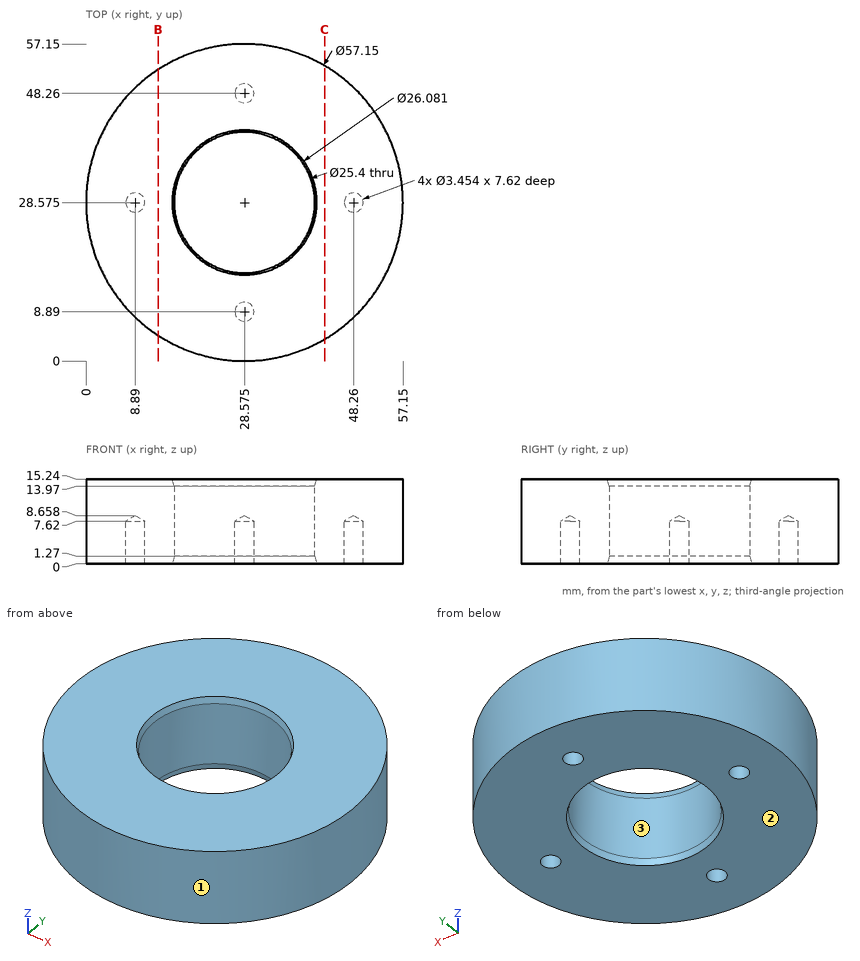
Here's the drawing with two shaded views (mm, measured from the low corner). I have some questions. Round coordinates to 2 decimals unless told otherwise and drop trailing zeros. Order: outer loops, then holes, each group sorted by start corner. A loop starts at its lowest first (then second) coordinate and runs counter-clockwise, first axis right, second up. Notation, with made-up numbers: (24.25, 19.25) -> (41.25, 19.25) arc R24 cw to (41.25, 42.25) -> close; hole circle Ø8 at (-3.5, -22). An arc over 180 degrees is marked (long way). Write each question's results on one line, items separated by ' | '. Start each with the question number.
Item 1: Thinking about a two-plate mould opening in Y: for the marked faces 1, 2 and 3, which applies, +Y half, -Y half, draft (parallel to the pull), parting line (faces both ways), or undercut?
Item 2: Please list where these lines run through material, in increasing order: L1, parallel to Y at x = 8.5, z = 6.5; L2, parallel to Y at x = 24, z = 7.75; L3, parallel to X at y = 48.26, z = 3.25.
Item 3: If we section it at B-B, the plane x = 13: Write out the boundary of the cut face in (y, z), then the cut area to 3 significant figures.
Item 4: If we section it at C-C, the plane x = 43: Write out the boundary of the cut face in (y, z).
Item 5: Will these pins go through, and if not, where does the flat tip stop? pin 1 (1 mm diameter, centred on y = 47.5, z = 9.5, fed in from +X) (1 decimal); pin 2 (1 mm diameter, centred on y = 34, z = 11.5, fed in from +X); pin 3 (2 mm diameter, centred on y = 38, z = 3.5, fed in from -X); pin 4 (20.5 mm diameter, centred on x = 28.575, y = 28.575, fed in from -Z).
Results:
1) face 1: parting line | face 2: draft | face 3: undercut
2) L1: y = 8.24 to 26.89, 30.26 to 48.91 | L2: y = 0.37 to 16.73, 40.42 to 56.78 | L3: x = 7.86 to 26.85, 30.3 to 49.29
3) outline: (4.62, 0) -> (52.53, 0) -> (52.53, 15.24) -> (4.62, 15.24) -> close | area: 730 mm2
4) outline: (3.91, 0) -> (53.24, 0) -> (53.24, 15.24) -> (3.91, 15.24) -> close
5) pin 1: stops at x = 50.4 | pin 2: stops at x = 56.72 | pin 3: stops at x = 1.27 | pin 4: passes through
